from build123d import *

# Parameters (mm, degrees)
SKETCH8_W               = 85
SKETCH8_H               = 10
BOSS_EXTRUDE4_DEPTH     = 10
SKETCH9_W               = 82
SKETCH9_H               = 9.9
BOSS_EXTRUDE5_DEPTH     = 10
CUT_EXTRUDE2_DEPTH      = 176.278228509
CUT_EXTRUDE2_DEPTH_BACK = 176.278228509
BOSS_EXTRUDE6_DEPTH     = 114


with BuildPart() as part:
    # Sketch8 → Boss-Extrude4 (new body)
    with BuildSketch(Plane(origin=(0, 0, 0), x_dir=(1, 0, 0), z_dir=(0, 1, 0))):
        with Locations((90.205142442, -69.45)):
            Rectangle(SKETCH8_W, SKETCH8_H)
    extrude(amount=BOSS_EXTRUDE4_DEPTH)


with BuildPart() as body_2:
    # Sketch9 → Boss-Extrude5 (new body)
    with BuildSketch(Plane(origin=(0, 87, 0), x_dir=(1, 0, 0), z_dir=(0, 1, 0))):
        with Locations((91.705142442, -32.5)):
            Rectangle(SKETCH9_W, SKETCH9_H)
    extrude(amount=-BOSS_EXTRUDE5_DEPTH)


    add(part.part)  # loft1 joins it to this body
    # loft from a face of the part (loft1)
    loft([body_2.faces().sort_by_distance((91.705142442, 77, 32.5))[0], body_2.faces().sort_by_distance((90.205142442, 10, 69.45))[0]])

    # Sketch1 → Cut-Extrude2 (cut, two sides)
    with BuildSketch(Plane.XY) as cut_extrude2_sk:
        Polygon((122.705142442, 87), (71.403683768, 87), (122.705142442, 58.6920409), align=None)
        Polygon((64.644486366, 10), (93.961994057, 63.13102594), (122.705142442, 47.270660759), (122.705142442, 10), align=None)
        Polygon((47.705142442, 0), (40.860670667, 0), (50.705142442, 87), (85.206484761, 67.96228426), align=None)
    extrude(amount=CUT_EXTRUDE2_DEPTH, mode=Mode.SUBTRACT)
    extrude(cut_extrude2_sk.sketch, amount=-CUT_EXTRUDE2_DEPTH_BACK, mode=Mode.SUBTRACT)

    # Sketch10 → Boss-Extrude6 (add)
    with BuildSketch(Plane(origin=(132.705142442, 0, 0), x_dir=(0, 0, -1), z_dir=(1, 0, 0))):
        Polygon((-64.55, 9.9), (-64.55, 0), (-74.45, 0), align=None)
    extrude(amount=-BOSS_EXTRUDE6_DEPTH)


solid = body_2.part
Work out the finished part from the listing and answer in its coordinate system (mm). A direction names the side the tool comes from. Coordinates: 2 decimals unless noted, no trailing zeros. Write each loop counter-clockwise with the first axis right and the second up, starting at its lowest first coordinate (ties: lowest second). Pieces come first, ordered by that corner, then holes.
1. The part is cut by section A-A, the plane x = 34. Write down the section's boundary in (y, z).
Results list:
outline: (0, 64.55) - (9.9, 64.55) - (0, 74.45) - close
2. The part is cut by section B-B, the plane x = 81.5. State how many separate pieces and enclosed holes the cut face has, and give its area (3 significant figures).
Results list:
separate pieces: 3
enclosed holes: 0
area: 419 mm2
3. Flat-ended cylindrical pins translate along their axes: pin 1 (3 mm diameter, centred on x = 82, y = 5.5, fed in from -Z); pin 2 (5 mm diameter, centred on x = 77.5, y = 83, fed in from +Z); pin 3 (11 mm diameter, centred on x = 105, z = 69, fed in from +Y). Find the tip coordinate at first contact, or state that the pin passes through.
Results list:
pin 1: stops at z = 64.45
pin 2: stops at z = 37.45
pin 3: stops at y = 10
4. For a pull along X with two mould halves and no side action, classify faces 1 (the flat face through (67.714, 77.614, 33.237)), 2 (the flat face through (108.132, 55.312, 44.397)), 3 (the flat face through (61, 87, 32)) as +X half, -X half, draft (parallel to the pull), parting line (faces both ways), or undercut.
Results list:
face 1: -X half
face 2: undercut
face 3: draft
5. For faces 4 (the flat face through (128, 82, 37.45)), 5 (the flat face through (36.18, 4.88, 69.57)), 6 (the flat face through (90, 5, 64.45)), determine the directions among +Z, -Z, +X, -X, +Y, -Y from which every point of the face is accessible in a straight line to the end or side of a thin tool.
Results list:
face 4: +Z, +X, -X, +Y
face 5: +Z, -X, +Y
face 6: -Z, +X, -X, -Y
6. Consider line 1 along X through (y, z) = (61, 42); line 2 along Z through (x, y) = (91.5, 8); line 3 along X through (y, z) = (16.5, 62). Determine where each line is inside the solid, lowest interval first.
Results list:
line 1: x = 81.36 to 92.79, 97.82 to 118.52, 122.71 to 132.71
line 2: z = 64.45 to 74.45
line 3: x = 56.81 to 68.23, 122.71 to 132.71
